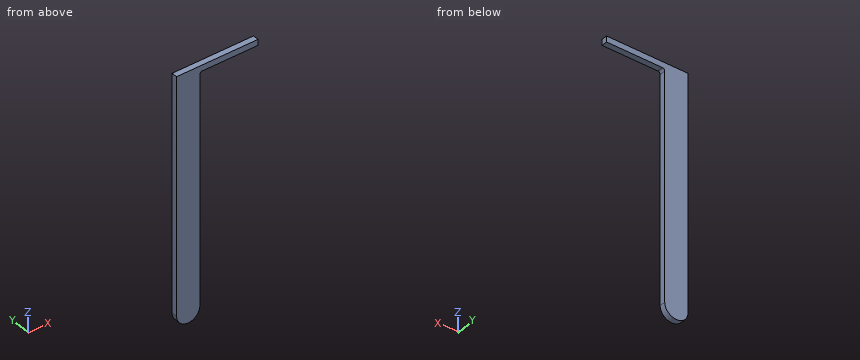
from build123d import *

# Parameters (mm, degrees)
BOSS_EXTRUDE1_DEPTH = 6.35
SKETCH2_W           = 88.9
SKETCH2_H           = 6.35
BOSS_EXTRUDE2_DEPTH = 6.35
FILLET1_R           = 2.54


with BuildPart() as part:
    # Sketch1 → Boss-Extrude1 (new body)
    with BuildSketch(Plane(origin=(0, 0, 0), x_dir=(1, 0, 0), z_dir=(0, 1, 0))):
        with BuildLine():
            ThreePointArc((12.7, 0), (0, -12.7), (-12.7, 0))
            Line((-12.7, 0), (-12.7, -247.65))
            Line((-12.7, -247.65), (12.7, -247.65))
            Line((12.7, -247.65), (12.7, 0))
        make_face()
        with BuildLine():
            ThreePointArc((12.7, 0), (0, 12.7), (-12.7, 0))
            Line((-12.7, 0), (12.7, 0))
        make_face()
        with BuildLine():
            Line((12.7, 0), (-12.7, 0))
            ThreePointArc((-12.7, 0), (0, -12.7), (12.7, 0))
        make_face()
    extrude(amount=BOSS_EXTRUDE1_DEPTH)

    # Sketch2 → Boss-Extrude2 (add)
    with BuildSketch(Plane(origin=(0, 6.35, 0), x_dir=(1, 0, 0), z_dir=(0, 1, 0))):
        with Locations((31.75, -250.825)):
            Rectangle(SKETCH2_W, SKETCH2_H)
    extrude(amount=-BOSS_EXTRUDE2_DEPTH)

    # Fillet1
    fillet1_edges = [part.edges().sort_by_distance(p)[0] for p in [
        (12.7, 3.175, 247.65),
    ]]
    fillet(fillet1_edges, radius=FILLET1_R)


solid = part.part
Geometry: final body of the model. Coordinates: model frame, mm. Round coordinates to 2 decimals unless told otherwise and drop trailing zeros. Order: outer loops, then holes, each group sorted by start corner. A loop starts at its lowest first (then second) coordinate and runs counter-clockwise, first axis right, second up. Notation, with made-up numbers: (-39.5, 27) -> (-0.5, 27) arc R13 ccw to (-0.5, 35) -> close; hole circle Ø1 at (53.5, 62). An arc over 180 degrees is marked (long way). Put each result on its own line as item: value. Start each with the question number.
Q1. Section B-B on x = 23.5. Return the cut outline in (y, z), and give its area (3 significant figures).
Q2. Section A-A on y = 3.5. Return the cut outline in (x, z), and give its area (3 significant figures).
Q3. Section C-C on z = 123. Return the cut outline in (x, y).
Q4. Line query: probe 1 along Z at (x, y) = (45, 2); probe 2 along X at (y, z) = (5, 44); probe 3 along Z at (x, y) = (-1, 2.5). Output: solid intervals per line, ascending.
Ans:
1. outline: (0, 247.65) -> (6.35, 247.65) -> (6.35, 254) -> (0, 254) -> close
1. area: 40.3 mm2
2. outline: (-12.7, 0) arc R12.7 ccw to (12.7, 0) -> (12.7, 245.11) arc R2.54 cw to (15.24, 247.65) -> (76.2, 247.65) -> (76.2, 254) -> (-12.7, 254) -> close
2. area: 7,110 mm2
3. outline: (-12.7, 0) -> (12.7, 0) -> (12.7, 6.35) -> (-12.7, 6.35) -> close
4. probe 1: z = 247.65 to 254
4. probe 2: x = -12.7 to 12.7
4. probe 3: z = -12.66 to 254
